Autodesk Inventor part; units mm, degrees
ref_plane "Work Plane1" through (11.5, 10, 0) normal (1, 0, 0) x (0, 1, 0)
ref_plane "Work Plane2" through (0, 10, -11.5) normal (0, 0, 1) x (1, 0, 0)
ref_plane "XZ Plane" through (0, 0, 0) normal (0, 1, 0) x (-1, 0, 0)
sketch "Sketch1" plane through (0, 0, 0) normal (0, 1, 0) x (-1, 0, 0)
  circle A0 centre (0, 0) radius 5
  circle A1 centre (0, 0) radius 14
  dimension "d0" = 10
  dimension "d1" = 28
extrude "Extrusion1" add sketch "Sketch1" along normal blind 10
sketch "Sketch2" plane through (0, 10, 0) normal (0, 1, 0) x (1, 0, 0)
  circle A0 centre (0, 0) radius 11.5
  circle A1 centre (0, 0) radius 5
  dimension "d4" = 23
extrude "Extrusion2" add sketch "Sketch2" along normal blind 10
fillet "Fillet1" radius 1 1 edges at (-11.5, 10, 0)
ref_plane "Work Plane1" through (11.5, 10, 0) normal (1, 0, 0) x (0, 1, 0)
fillet "Fillet2" radius 1 1 edges at (-11.5, 20, 0)
ref_plane "Work Plane2" through (0, 10, -11.5) normal (0, 0, 1) x (1, 0, 0)
sketch "Sketch4" plane through (0, 10, -11.5) normal (0, 0, 1) x (1, 0, 0)
  line L0 (-10.5, 10) -> (10.5, 10)
  point P0 (0, -10)
  point P1 (0, 5)
  dimension "d21" = 5
  dimension "d22" = 0
sketch "Sketch3" plane through (11.5, 10, 0) normal (1, 0, 0) x (0, 1, 0)
  line L0 (10, -11.5) -> (10, 11.5)
  point P0 (-10, 0)
  point P1 (5, 0)
  dimension "d8" = 5
  dimension "d9" = 0
hole "Hole1" at (11.5, 15, 0) direction (-1, 0, 0) diameter 3.242 end up to surface
hole "Hole2" at (0, 15, -11.5) direction (0, 0, 1) diameter 3.242 end up to surface
sketch "Sketch5" plane through (0, 20, 0) normal (0, 1, 0) x (1, 0, 0)
  line L0 (-2, 4.5826) -> (2, 4.5826)
  line L1 (2, 4.5826) -> (2, 6.8)
  line L2 (2, 6.8) -> (-2, 6.8)
  line L3 (-2, 6.8) -> (-2, 4.5826)
  circle A0 centre (0, 0) radius 5
  dimension "d30" = 4
  dimension "d31" = 6.8
extrude "Extrusion3" cut sketch "Sketch5" against normal through all contours A0 L0 | L3 L2 L1 A0 picked at (0.3405, 4.6866)
chamfer "Chamfer2" distance 0.5 angle 45 8 edges at (-2, 20, -5.6913) (0, 20, -6.8) (2, 20, -5.6913) (0, 20, 5) (0, 0, -6.8) (-2, 0, -5.6913) (2, 0, -5.6913) (0, 0, 5)
sketch "Sketch6" plane through (0, 0, 0) normal (0, -1, 0) x (1, 0, 0)
  circle A0 centre (0, 0) radius 15
  dimension "d37" = 30
sketch "Sketch7" plane through (0, 10, 0) normal (0, 1, 0) x (1, 0, 0)
  circle A0 centre (0, 0) radius 15
  dimension "d38" = 30
properties part number "gear_khk_SUS1-28J10" material "Steel, High Strength, Low Alloy"
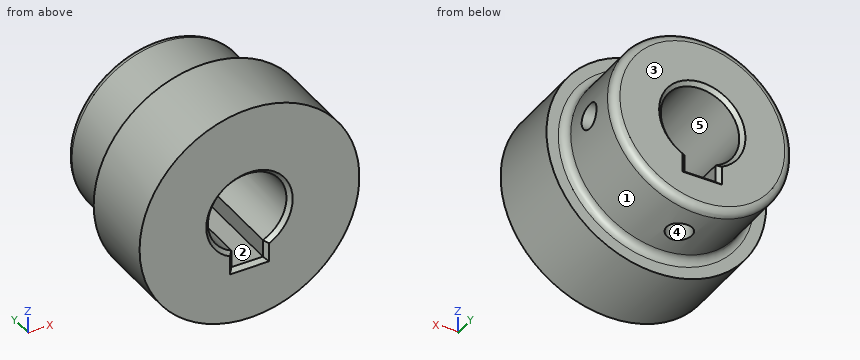
Geometry check sheet. Reference: the model listing, model coordinates, mm. Face numbers are marked on the shaded views. A direction names the side the tool comes from. Round coordinates to 2 decimals unless told otherwise and drop trailing zeros. Order: outer loops, then holes, each group sorted by start corner. A loop starts at its lowest first (then second) coordinate and runs counter-clockwise, first axis right, second up. Notation, with made-up numbers: M -30,76.25 L -13,76.25 A25 ccw -13,96.25 Z; hole C 5.25,39 d1. An arc over 180 degrees is marked long. Answer in a Markdown table with one row per item. Add a question column.
Item 1: Sectioned sample at A-A, the plane z = 0. Enter the section's corners in (x, y).
Item 2: Material ranges on L1, parallel to X at y = 17, z = -0.25; L2, parallel to Y at x = 7.5, z = 0; L3, parallel to Z at x = 0, y = 6, recorded low to high. Write a range as [from, to].
Item 3: Set-up check for the marked faces 4 and 5: record each of +Z, -Z, +X, -X, +Y, -Y from which the full face is reachable in a straight line by a thin tool's end or side.
Item 4: Sectioned sample at C-C, the plane y = 5.75. Enter the section's corners in (x, z), plus the area to 3 significant figures.
Item 5: Sectioned sample at D-D, the plane y = 13. Enter the section's corners in (x, z).
Item 6: Sectioned sample at B-B, the plane x = 0. Enter the section's corners in (y, z), plus the area to 3 significant figures.
Item 7: Draft check along X on the marked faces 1, 2 and 3. Enter one of: released by +X, released by -X, zero draft, split by the parting line, or undercut.
Item 8: Depth check by flat-ended pin: pin 1 Ø2 at (y, z) = (17, 3) entering from +X; pin 2 Ø4 at (y, z) = (9, -10) entering from -X; pin 3 Ø2 at (x, z) = (4, -1) entering from +Y; pin 4 Ø12 at (x, y) = (5, 12.5) entering from -Z. Enter the tip coordinate at first touch or a pass-through.
Filled in:
| question | item | result |
|---|---|---|
| 1 | outline | M -14,0 L -5.5,0 L -5,0.5 L -5,19.5 L -5.5,20 L -10.5,20 A1 ccw -11.5,19 L -11.5,11 A1 cw -12.5,10 L -14,10 Z; M 5,0.5 L 5.5,0 L 14,0 L 14,10 L 12.5,10 A1 cw 11.5,11 L 11.5,13.38 L 5,13.38 Z; M 5,16.62 L 11.5,16.62 L 11.5,19 A1 ccw 10.5,20 L 5.5,20 L 5,19.5 Z |
| 2 | L1 | x = [-11.5, -4.99], [4.99, 11.5] |
| 2 | L2 | y = [0, 13.38], [16.62, 20] |
| 2 | L3 | z = [-14, -6.8], [5, 14] |
| 3 | face 4 | -Z |
| 3 | face 5 | +Y, -Y |
| 4 | outline | C 0,0 d28; hole M -2,-6.8 L 2,-6.8 L 2,-4.58 A5 ccw long -2,-4.58 Z |
| 4 | area | 529 mm² |
| 5 | outline | C 0,0 d23; hole M -2,-6.8 L 2,-6.8 L 2,-4.58 A5 ccw long -2,-4.58 Z |
| 6 | outline | M 0,-14 L 10,-14 L 10,-12.5 A1 cw 11,-11.5 L 13.38,-11.5 L 13.38,-6.8 L 0.5,-6.8 L 0,-7.3 Z; M 0,5.5 L 0.5,5 L 19.5,5 L 20,5.5 L 20,10.5 A1 ccw 19,11.5 L 11,11.5 A1 cw 10,12.5 L 10,14 L 0,14 Z; M 16.62,-11.5 L 19,-11.5 A1 ccw 20,-10.5 L 20,-7.3 L 19.5,-6.8 L 16.62,-6.8 Z |
| 6 | area | 258 mm² |
| 7 | face 1 | split by the parting line |
| 7 | face 2 | undercut |
| 7 | face 3 | zero draft |
| 8 | pin 1 | stops at x = 11.32 |
| 8 | pin 2 | stops at x = -11.49 |
| 8 | pin 3 | stops at y = 19.62 |
| 8 | pin 4 | stops at z = -14 |
